from build123d import *

# Parameters (mm, degrees)
SKETCH3_R           = 10
BOSS_EXTRUDE1_DEPTH = 750
SKETCH6_R           = 15
BOSS_EXTRUDE2_DEPTH = 1
BOSS_EXTRUDE3_START = 20
SKETCH7_R           = 10
BOSS_EXTRUDE3_DEPTH = 20
SKETCH8_W           = 65
SKETCH8_H           = 6
CUT_EXTRUDE1_DEPTH  = 6


with BuildPart() as part:
    # Sketch3 → Boss-Extrude1 (new body)
    with BuildSketch(Plane(origin=(0, 0, 0), x_dir=(0, 0, -1), z_dir=(1, 0, 0))):
        Circle(SKETCH3_R)
    extrude(amount=BOSS_EXTRUDE1_DEPTH)

    # Loft1: read off the stored shape, not the designer's step
    # Loft1: loft between two sections, ruled curve by curve
    loft1_from = [
        Edge.make_bspline([(130, 13.420275273, -6.700463537), (130, 0.019348199, -33.541014082), (130, -26.821202346, -20.140087008), (130, -13.420275273, 6.700463537), (130, -0.019348199, 33.541014082), (130, 26.821202346, 20.140087008), (130, 13.420275273, -6.700463537)], [0, 0, 0, 0, 0.5, 0.5, 0.5, 1, 1, 1, 1], 3, [1, 0.333333333, 0.333333333, 1, 0.333333333, 0.333333333, 1]),
    ]
    loft1_to = [
        Edge.make_bspline([(110, 7.764671539, -9.149310132), (110, -10.533948725, -24.67865321), (110, -26.063291803, -6.380032946), (110, -7.764671539, 9.149310132), (110, 10.533948725, 24.67865321), (110, 26.063291803, 6.380032946), (110, 7.764671539, -9.149310132)], [0, 0, 0, 0, 0.5, 0.5, 0.5, 1, 1, 1, 1], 3, [1, 0.333333333, 0.333333333, 1, 0.333333333, 0.333333333, 1]),
    ]
    loft1 = Solid(Shell([*[Face.make_surface_from_curves(loft1_from[k], loft1_to[k]) for k in range(1)], Face(Wire(loft1_from)), Face(Wire(loft1_to))]))
    add(loft1)

    # Sketch6 → Boss-Extrude2 (add)
    with BuildSketch(Plane(origin=(500, 0, 0), x_dir=(0, 0, -1), z_dir=(1, 0, 0))):
        Circle(SKETCH6_R)
    extrude(amount=BOSS_EXTRUDE2_DEPTH)

    # Sketch7 → Boss-Extrude3 (add)
    with BuildSketch(Plane.ZY.offset(BOSS_EXTRUDE3_START)):
        with Locations(Location((0, 0, 0), (0, 0, 180))):
            Circle(SKETCH7_R)
    extrude(amount=-BOSS_EXTRUDE3_DEPTH)

    # Sketch8 → Cut-Extrude1 (cut)
    with BuildSketch(Plane(origin=(0, 12.5, 0), x_dir=(1, 0, 0), z_dir=(0, 1, 0))):
        with Locations((162.5, 0)):
            Rectangle(SKETCH8_W, SKETCH8_H)
    extrude(amount=-CUT_EXTRUDE1_DEPTH, mode=Mode.SUBTRACT)


solid = part.part
Build history of the part. All positions in model axes, mm. A direction names the side the tool comes from. Coordinates: 2 decimals unless noted, no trailing zeros. Write each loop counter-clockwise with the first axis right and the second up, starting at its lowest first coordinate (ties: lowest second). Pieces come first, ordered by that corner, then holes.
(1) Drill centre lines: line 1 (X direction, y = 8.5, z = -2.5); line 2 (X direction, y = 10.5, z = -4.5); line 3 (Y direction, x = 656.5, z = -1.5). Where is each one in solid material? Low to high.
(2) Pin check, flat tips, straight feed: pin 1 Ø0.9 at (x, y) = (156, 7.5) entering from +Z; pin 2 Ø6 at (x, y) = (336, -4) entering from +Z; pin 3 Ø1.5 at (y, z) = (11, 0.5) entering from +X. Stop position of each tip, or through.
(3) Mould opens along X. For faces 1 (the flat face through (500, -10, -3)), 2 (the cylindrical face through (312.41, -9.76, 2.17)), 3 (the flat face through (-20, 0, 0)), 4 (the cylindrical face through (623.76, -9.76, 2.17)) say: pulls with the +X half, pulls with the -X half, needs draft (parallel to the pull), parting line crosses it, or undercut.
(4) 3-axis set-ups, long thin cutter, end or side, ignore diameter. For faces 5 (the flat face through (110, -10, -4)), 6 (the flat face through (750, 0, 0)), 7 (the flat face through (501, -10, -3)): which of +Z, -Z, +X, -X, +Y, -Y reach the whole face in a straight line?
(5) Cut at A-A on x = 27. List the corners of the cut face in (y, z), and give its area (3 significant figures).
Working result:
1. line 1: x = -20 to 130, 195 to 750
1. line 2: x = 110 to 130, 500 to 501
1. line 3: y = -9.89 to 9.89
2. pin 1: stops at z = 7.09
2. pin 2: stops at z = 9.95
2. pin 3: stops at x = 501
3. face 1: undercut
3. face 2: undercut
3. face 3: pulls with the -X half
3. face 4: needs draft
4. face 5: -X
4. face 6: +Z, -Z, +X, +Y, -Y
4. face 7: +X
5. outline: circle Ø20 at (0, 0)
5. area: 314 mm2
